Autodesk Inventor part; units mm, degrees
ref_plane "YZ Plane" through (0, 0, 0) normal (1, 0, 0) x (0, 1, 0)
ref_plane "XZ Plane" through (0, 0, 0) normal (0, 1, 0) x (-1, 0, 0)
ref_plane "XY Plane" through (0, 0, 0) normal (0, 0, 1) x (1, 0, 0)
sketch "Sketch1" plane through (0, 0, 0) normal (0, 1, 0) x (-1, 0, 0)
  line L0 (34.4209, 32.9812) -> (-34.1591, 32.9812)
  line L1 (-34.1591, 32.9812) -> (-34.1591, -20.6128)
  line L2 (-34.1591, -20.6128) -> (34.4209, -20.6128)
  line L3 (34.4209, -20.6128) -> (34.4209, 32.9812)
  circle A0 centre (19.6889, 30.9492) radius 1.524
  circle A1 centre (19.6889, -17.3108) radius 1.524
  circle A2 centre (-31.1111, -14.0088) radius 1.524
  circle A3 centre (-31.1111, 13.9312) radius 1.524
  point P0 (0, 0)
  dimension "d0" = 68.58
  dimension "d1" = 53.594
  dimension "d2" = 14.732
  dimension "d3" = 2.032
  dimension "d4" = 3.048
  dimension "d5" = 48.26
  dimension "d6" = 6.604
  dimension "d7" = 3.048
  dimension "d8" = 27.94
extrude "Extrusion1" add sketch "Sketch1" along normal blind 2.54
properties part number "arduino uno model"
CAD build for the part. Positions are in the model's coordinates, mm. Give positions to 0.01 mm unless a question says otherwise; leave off trailing zeros. Order: outer loops, then holes, each group sorted by start corner. A loop starts at its lowest first (then second) coordinate and runs counter-clockwise, first axis right, second up. Notation, with made-up numbers: M 40,51 L 67,51 A10 cw 67,66 Z; hole C 73.25,39 d3. An arc over 180 degrees is marked long. Put each result on its own line as item: value. Start each with the question number.
(1) Drill centre lines: line 1 along Z through (x, y) = (-19.5, 1); line 2 along X through (y, z) = (1.15, 13); line 3 along X through (y, z) = (1.75, -14.5). Where is each one in solid material? Low to high.
(2) Mould opens along X. For faces 1 (the flat face through (0, 0, 7)), 2 (the flat face through (34.159, 1, 7)), 3 (the cylindrical face through (-19.49, 1.25, 29.44)) say: +X half, -X half, draft (parallel to the pull), parting line (faces both ways), or undercut.
(3) Flat gauge pin, fed straight in: pin 1 Ø1.8 at (x, z) = (31.11, -14.01) entering from -Y. Where does the tip first touch, or does it go through?
(4) Saw through at A-A, the plane z = -16.5. Write the cut outline in (x, y), then the cut area to 3 significant figures.
Check result:
1. line 1: z = -20.61 to -18.82, -15.8 to 29.44, 32.46 to 32.98
1. line 2: x = -34.42 to 29.9, 32.32 to 34.16
1. line 3: x = -34.42 to 29.67, 32.55 to 34.16
2. face 1: draft
2. face 2: +X half
2. face 3: undercut
3. pin 1: passes through
4. outline: M -34.42,0 L -20.98,0 L -20.98,2.54 L -34.42,2.54 Z; M -18.4,0 L 34.16,0 L 34.16,2.54 L -18.4,2.54 Z
4. area: 168 mm2
